from build123d import *

# Parameters (mm, degrees)
BOSS_EXTRUDE1_DEPTH  = 55
BOSS_EXTRUDE2_START  = -5
SKETCH3_W            = 10
SKETCH3_H            = 10
BOSS_EXTRUDE2_DEPTH  = 8
M4_CLEARANCE_HOLE1_D = 4.5
FILLET2_R            = 10
FILLET3_R            = 1


with BuildPart() as part:
    # Sketch2 → Boss-Extrude1 (new, symmetric)
    with BuildSketch(Plane(origin=(0, 0, 0), x_dir=(1, 0, 0), z_dir=(0, 1, 0))):
        Polygon((0, 0), (20, 0), (20, -10), (10, -10), (10, -20), (0, -20), align=None)
    extrude(amount=BOSS_EXTRUDE1_DEPTH, both=True)

    # Sketch3 → Boss-Extrude2 (add)
    with BuildSketch(Plane(origin=(0, 55, 0), x_dir=(1, 0, 0), z_dir=(0, 1, 0)).offset(BOSS_EXTRUDE2_START)):
        with Locations((15, -15)):
            Rectangle(SKETCH3_W, SKETCH3_H)
    boss_extrude2 = extrude(amount=BOSS_EXTRUDE2_DEPTH)

    # M4 Clearance Hole1 (through all)
    with Locations(Plane(origin=(15, 50, 15), x_dir=(0, 0, -1), z_dir=(0, -1, 0))):
        with Locations((0, 0)):
            m4_clearance_hole1 = Hole(M4_CLEARANCE_HOLE1_D / 2)

    # Mirror1: Boss-Extrude2, M4 Clearance Hole1 across plane
    add(boss_extrude2.mirror(Plane.ZX))
    add(m4_clearance_hole1.mirror(Plane.ZX), mode=Mode.SUBTRACT)

    # Fillet2
    fillet2_edges = [part.edges().sort_by_distance(p)[0] for p in [
        (0, 0, 0),
    ]]
    fillet(fillet2_edges, radius=FILLET2_R)

    # Fillet3
    fillet3_edges = [part.edges().sort_by_distance(p)[0] for p in [
        (15, 55, 0),
        (0, -55, 15),
        (0, 55, 15),
        (2.928932188, -55, 2.928932188),
        (2.928932188, 55, 2.928932188),
        (15, -55, 0),
    ]]
    fillet(fillet3_edges, radius=FILLET3_R)


solid = part.part
Geometry check sheet. Reference: the model listing, model coordinates, mm. A direction names the side the tool comes from. Round coordinates to 2 decimals unless told otherwise and drop trailing zeros. Write each loop counter-clockwise with the first axis right and the second up, starting at its lowest first coordinate (ties: lowest second). Pieces come first, ordered by that corner, then holes. Notation, with made-up numbers: (60.5, -35.75) -> (83.5, -35.75) arc R17 ccw to (83.5, -23.75) -> close; hole circle Ø5 at (-19.75, 18.25). An arc over 180 degrees is marked (long way). One line per item, written item: value. Start each with the question number.
(1) Go/stop test with flat-tipped pins: pin 1 Ø2.5 at (x, z) = (15, 15) entering from +Y; pin 2 Ø12 at (x, y) = (2.5, -44.5) entering from -Z; pin 3 Ø8 at (x, y) = (17.5, 4) entering from +Z; pin 4 Ø1.5 at (y, z) = (-42, 8) entering from -X. Record where each tip stops, or that it passes through.
(2) Draft check along Y on faces 6 (the flat face through (12.7, 50, 13.8)), 7 (the flat face through (12.7, 58, 13.8)), 8 (the flat face through (10, 56, 15)). Enter one of: +Y half, -Y half, draft (parallel to the pull), parting line (faces both ways), or undercut.
(3) Scan lines: line 1 (Z direction, x = 15, y = -52.5); line 2 (X direction, y = -56.25, z = 15). Record each from-to range of solid material in increasing order. Write a range as [from, to].
(4) Cross-section at B-B, the plane x = 15. Record the cut outline in (y, z).
(5) Access from +Z, -Z, +X, -X, +Y, -Y to the whole of each face (thin tool, end or side, straight path). Record for faces 1 (the flat face through (12.7, -58, 13.8)), 2 (the flat face through (15, -56, 10)), 3 (the flat face through (12.7, -50, 13.8)), 4 (the flat face through (15, 56, 10)), 5 (the flat face through (10, -56, 15)).
(6) Cross-section at A-A, the plane z = 15. Record the cut outline in (x, y).
(7) Cross-section at C-C, the plane y = 37. Record the cut outline in (x, z), and give its area (3 significant figures).
Answer:
1. pin 1: through
1. pin 2: z = 0.11
1. pin 3: z = 10
1. pin 4: x = 0.08
2. face 6: undercut
2. face 7: +Y half
2. face 8: draft
3. line 1: [0, 12.75], [17.25, 20]
3. line 2: [10, 12.75], [17.25, 20]
4. outline: (-58, 10) -> (-55, 10) -> (-55, 1) arc R1 ccw to (-54, 0) -> (54, 0) arc R1 ccw to (55, 1) -> (55, 10) -> (58, 10) -> (58, 12.75) -> (50, 12.75) -> (50, 10) -> (-50, 10) -> (-50, 12.75) -> (-58, 12.75) -> close; (-58, 17.25) -> (-50, 17.25) -> (-50, 20) -> (-58, 20) -> close; (50, 17.25) -> (58, 17.25) -> (58, 20) -> (50, 20) -> close
5. face 1: +Z, -Z, +X, -X, -Y
5. face 2: -Z, +X, -X, -Y
5. face 3: +Z, +X
5. face 4: -Z, +X, -X, +Y
5. face 5: +Z, -Z, -X, -Y
6. outline: (0, -54) arc R1 ccw to (1, -55) -> (10, -55) -> (10, -58) -> (12.75, -58) -> (12.75, -50) -> (10, -50) -> (10, 50) -> (12.75, 50) -> (12.75, 58) -> (10, 58) -> (10, 55) -> (1, 55) arc R1 ccw to (0, 54) -> close; (17.25, -58) -> (20, -58) -> (20, -50) -> (17.25, -50) -> close; (17.25, 50) -> (20, 50) -> (20, 58) -> (17.25, 58) -> close
7. outline: (0, 10) arc R10 ccw to (10, 0) -> (20, 0) -> (20, 10) -> (10, 10) -> (10, 20) -> (0, 20) -> close
7. area: 279 mm²
